Part model, mm, in its own coordinate system. A direction names the side the tool comes from. Give positions to 0.01 mm unless a question says otherwise; leave off trailing zeros. Loops run counter-clockwise (first coordinate to the right, second up) from the corner with the lowest first, then second, coordinate; pieces in that order, holes last. Notation, with made-up numbers: M 55,43.25 L 102,43.25 A19 ccw 102,64.25 Z; hole C -39.5,-37 d6. An arc over 180 degrees is marked long. Answer in a Markdown table with one row per item.
from build123d import *

# Parameters (mm, degrees)
SKETCH1_W                = 2438.4
SKETCH1_H                = 1219.2
BOSS_EXTRUDE1_DEPTH      = 102
EXTRUDE_THIN1_DEPTH      = 26
EXTRUDE_THIN1_DEPTH_BACK = 24
BOSS_EXTRUDE2_DEPTH      = 0.17


with BuildPart() as part:
    # Sketch1 → Boss-Extrude1 (new body)
    with BuildSketch(Plane(origin=(0, 0, 0), x_dir=(1, 0, 0), z_dir=(0, 1, 0))):
        with Locations((1219.2, 609.6)):
            Rectangle(SKETCH1_W, SKETCH1_H)
    extrude(amount=BOSS_EXTRUDE1_DEPTH)

    # Sketch2 → Extrude-Thin1 (add, two sides)
    with BuildSketch(Plane(origin=(0, 102, 0), x_dir=(1, 0, 0), z_dir=(0, 1, 0))) as extrude_thin1_sk:
        Polygon((0, 0), (2133.6, 0), (2438.4, 457.2), (2438.4, 762), (2133.6, 1219.2), (0, 1219.2), (0, 1231.2), (2140.022205102, 1231.2), (2450.4, 765.633307653), (2450.4, 453.566692347), (2140.022205102, -12), (0, -12), align=None)
    extrude(amount=EXTRUDE_THIN1_DEPTH)
    extrude(extrude_thin1_sk.sketch, amount=-EXTRUDE_THIN1_DEPTH_BACK)

    # Sketch3 → Boss-Extrude2 (add)
    with BuildSketch(Plane(origin=(0, 102, 0), x_dir=(1, 0, 0), z_dir=(0, 1, 0))):
        Polygon((2400.4, 618.6), (611.985938124, 618.6), (611.985938124, 684.6), (593.985938124, 684.6), (593.985938124, 534.6), (611.985938124, 534.6), (611.985938124, 600.6), (2400.4, 600.6), (2117.8, 318), (611.985938124, 318), (611.985938124, 384), (593.985938124, 384), (593.985938124, 234), (611.985938124, 234), (611.985938124, 300), (2125.255844123, 300), (2418.4, 593.144155877), (2418.4, 626.055844123), (2125.255844123, 919.2), (611.985938124, 919.2), (611.985938124, 985.2), (593.985938124, 985.2), (593.985938124, 835.2), (611.985938124, 835.2), (611.985938124, 901.2), (2117.8, 901.2), align=None)
    extrude(amount=BOSS_EXTRUDE2_DEPTH)


solid = part.part
(1) Which spindle directions (+Z, -Z, +X, -X, +Y, -Y) get a long thin tool onto all of the face, cutting with end or side? Do faces 4 (the face through (2450.4, 103, -612)), 5 (the face through (2356, 102, -1101)), 6 (the face through (2288.134, 114.818, -987.4)). Say none if no direction does.
Recorded:
| item | result |
|---|---|
| face 4 | +Z, -Z, +X, +Y, -Y |
| face 5 | -Z, +X, +Y |
| face 6 | -X, +Y |
(2) Saw through at C-C (x = 833). Write the cut outline in (y, z), plus the area to 3 significant figures.
Recorded:
| item | result |
|---|---|
| outline | M 0,-1219.2 L 78,-1219.2 L 78,-1231.2 L 128,-1231.2 L 128,-1219.2 L 102,-1219.2 L 102,-919.2 L 102.17,-919.2 L 102.17,-901.2 L 102,-901.2 L 102,-618.6 L 102.17,-618.6 L 102.17,-600.6 L 102,-600.6 L 102,-318 L 102.17,-318 L 102.17,-300 L 102,-300 L 102,0 L 128,0 L 128,12 L 78,12 L 78,0 L 0,0 Z |
| area | 126,000 mm^2 |
(3) Saw through at B-B (z = -560.5). Write the cut outline in (x, y).
Recorded:
| item | result |
|---|---|
| outline | M 0,0 L 2438.4,0 L 2438.4,78 L 2450.4,78 L 2450.4,128 L 2438.4,128 L 2438.4,102 L 2385.76,102 L 2385.76,102.17 L 2360.3,102.17 L 2360.3,102 L 611.99,102 L 611.99,102.17 L 593.99,102.17 L 593.99,102 L 0,102 Z |
(4) Pull direction Y, two halves, no side cores. Call faces 1 (the face through (1202, 0, -618)), 2 (the face through (2293.038, 114.461, -1001.676)), 3 (the face through (2356, 102, -124)): +Y half, -Y half, draft (parallel to the pull), parting line (faces both ways), or undercut.
Recorded:
| item | result |
|---|---|
| face 1 | -Y half |
| face 2 | draft |
| face 3 | +Y half |
(5) Pin check, flat tips, straight feed: pin 1 Ø4 at (x, y) = (581, 53.5) entering from +Z; pin 2 Ø2 at (x, y) = (1619.5, 23.5) entering from -Z; pin 3 Ø2 at (x, z) = (695, -1083) entering from +Y. Stop position of each tip, or through.
Recorded:
| item | result |
|---|---|
| pin 1 | stops at z = 0 |
| pin 2 | stops at z = -1219.2 |
| pin 3 | stops at y = 102 |
(6) Saw through at A-A (x = 185.5). Write the cut outline in (y, z).
Recorded:
| item | result |
|---|---|
| outline | M 0,-1219.2 L 78,-1219.2 L 78,-1231.2 L 128,-1231.2 L 128,-1219.2 L 102,-1219.2 L 102,0 L 128,0 L 128,12 L 78,12 L 78,0 L 0,0 Z |
(7) Drill centre lines: line 1 along Z through (x, y) = (274, 104); line 2 along X through (y, z) = (87, -814); line 3 along Z through (x, y) = (1303.5, 70). Where is each one in solid material? Low to high.
Recorded:
| item | result |
|---|---|
| line 1 | z = -1231.2 to -1219.2, 0 to 12 |
| line 2 | x = 0 to 2438.4 |
| line 3 | z = -1219.2 to 0 |
(8) Saw through at D-D (z = -1069.5). Write the cut outline in (x, y), plus the area to 3 significant figures.
Recorded:
| item | result |
|---|---|
| outline | M 0,0 L 2438.4,0 L 2438.4,102 L 2247.82,102 L 2247.82,128 L 2233.4,128 L 2233.4,102 L 0,102 Z |
| area | 249,000 mm^2 |
